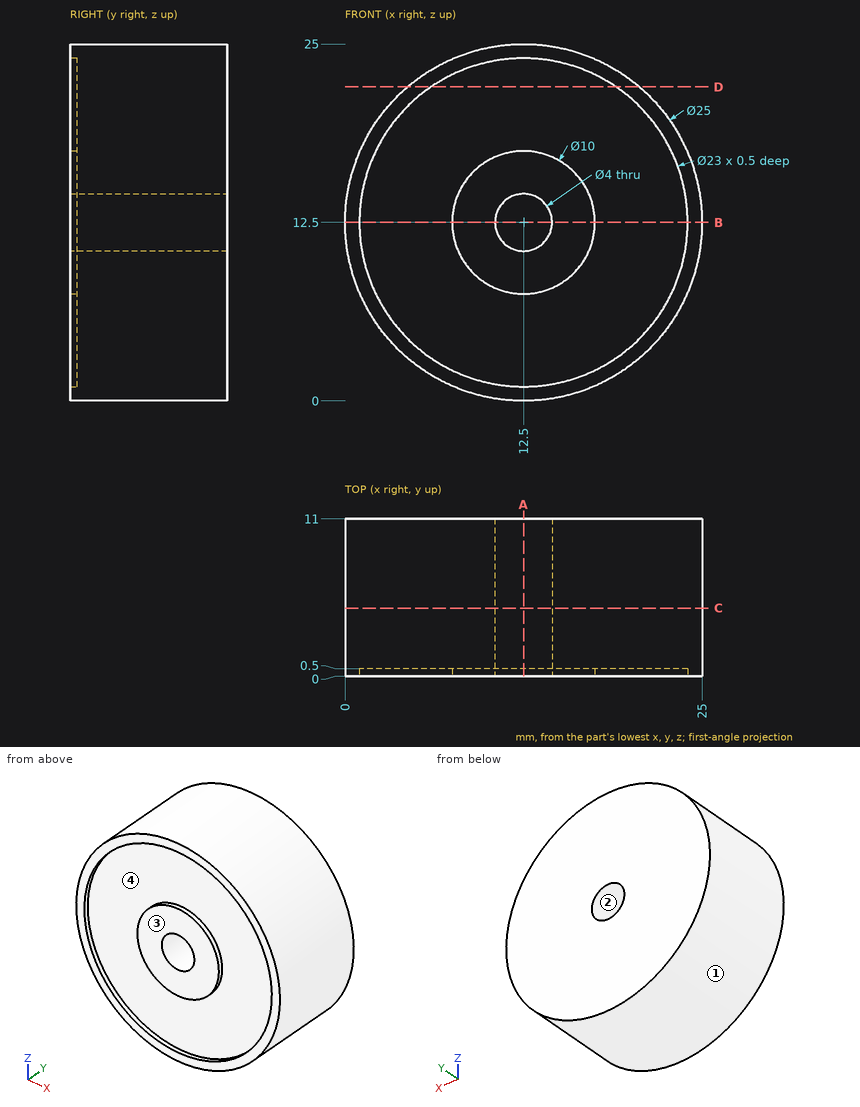
Can you work these out from the drawing? Everything is in mm from the part's minimum corner. Coordinates: 2 decimals unless noted, no trailing zeros. Order: outer loops, then holes, each group sorted by start corner. A loop starts at its lowest first (then second) coordinate and runs counter-clockwise, first axis right, second up. Notation, with made-up numbers: M -34,66.5 L -5,66.5 A24 cw -5,76.5 Z; hole C 1.25,52.5 d9. An arc over 180 degrees is marked long. Answer as CSV lines item,"result". Start each with the question number.
1. I want a section at B-B, the plane z = 12.5. Write out the boundary of the cut face in (x, y).
2. For pin 1 (5 mm diameter, centred on y = 2, z = 6, fed in from +X), with a flat end and sliding along its axis, tell me the tip position at first contact or that it passes through.
3. I want a section at D-D, the plane z = 22. Write out the boundary of the cut face in (x, y), and give its area (3 significant figures).
4. I want a section at A-A, the plane x = 12.5. Write out the boundary of the cut face in (y, z).
5. I need wall thicknesses on line 1 (X direction, y = 0.3, z = 12.5); line 2 (X direction, y = 4.25, z = 12.5); line 3 (Y direction, x = 20, z = 9). Which ranges of each line are inside material? Lowest first, please. Write a range as [from, to].
6. We'd pull the mould along Z, two halves only. Please class the marked faces 1, 2, 3 and 4: released by +Z, released by -Z, zero draft, split by the parting line, or undercut.
7. I want a section at C-C, the plane y = 4.75. Write out the boundary of the cut face in (x, z), and give its area (3 significant figures).
Recorded:
1,outline,"M 0,0 L 1,0 L 1,0.5 L 7.5,0.5 L 7.5,0 L 10.5,0 L 10.5,11 L 0,11 Z; M 14.5,0 L 17.5,0 L 17.5,0.5 L 24,0.5 L 24,0 L 25,0 L 25,11 L 14.5,11 Z"
2,pin 1,"stops at x = 24.34"
3,outline,"M 4.38,0 L 6.02,0 L 6.02,0.5 L 18.98,0.5 L 18.98,0 L 20.62,0 L 20.62,11 L 4.38,11 Z"
3,area,"172 mm2"
4,outline,"M 0,0 L 11,0 L 11,10.5 L 0,10.5 L 0,7.5 L 0.5,7.5 L 0.5,1 L 0,1 Z; M 0,14.5 L 11,14.5 L 11,25 L 0,25 L 0,24 L 0.5,24 L 0.5,17.5 L 0,17.5 Z"
5,line 1,"x = [0, 1], [7.5, 10.5], [14.5, 17.5], [24, 25]"
5,line 2,"x = [0, 10.5], [14.5, 25]"
5,line 3,"y = [0.5, 11]"
6,face 1,"split by the parting line"
6,face 2,"undercut"
6,face 3,"zero draft"
6,face 4,"undercut"
7,outline,"C 12.5,12.5 d25; hole C 12.5,12.5 d4"
7,area,"478 mm2"
